Geometry check sheet. Reference: the model listing, model coordinates, mm. Face numbers are marked on the shaded views. Coordinates: 2 decimals unless noted, no trailing zeros. Loops run counter-clockwise (first coordinate to the right, second up) from the corner with the lowest first, then second, coordinate; pieces in that order, holes last.
from build123d import *

# Parameters (mm, degrees)
SKETCH1_R           = 29
SKETCH1_R_2         = 25.5
BOSS_EXTRUDE1_DEPTH = 30
CUT_EXTRUDE1_START  = -4
SKETCH2_R           = 26.983908251
SKETCH2_R_2         = 25.5
CUT_EXTRUDE1_DEPTH  = 4
BOSS_EXTRUDE2_START = 6
SKETCH3_R           = 29
BOSS_EXTRUDE2_DEPTH = 6
SKETCH4_R           = 4
CUT_EXTRUDE2_DEPTH  = 4.3
SKETCH5_R           = 25.5
SKETCH5_R_2         = 25.1
BOSS_EXTRUDE3_DEPTH = 2


with BuildPart() as part:
    # Sketch1 → Boss-Extrude1 (new body)
    with BuildSketch(Plane(origin=(0, 0, 0), x_dir=(1, 0, 0), z_dir=(0, 1, 0))):
        with Locations(Location((0, 0, 0), (0, 0, 270))):
            Circle(SKETCH1_R)
        with Locations(Location((0, 0, 0), (0, 0, 270))):
            Circle(SKETCH1_R_2, mode=Mode.SUBTRACT)
    extrude(amount=BOSS_EXTRUDE1_DEPTH)

    # Sketch2 → Cut-Extrude1 (cut)
    with BuildSketch(Plane(origin=(0, 30, 0), x_dir=(1, 0, 0), z_dir=(0, 1, 0)).offset(CUT_EXTRUDE1_START)):
        with Locations(Location((0, 0, 0), (0, 0, 270))):
            Circle(SKETCH2_R)
        with Locations(Location((0, 0, 0), (0, 0, 270))):
            Circle(SKETCH2_R_2, mode=Mode.SUBTRACT)
    extrude(amount=CUT_EXTRUDE1_DEPTH, mode=Mode.SUBTRACT)

    # Fillet1: read off the stored shape, not the designer's step
    # Fillet1 outline → Fillet1 (revolve, cut)
    with BuildSketch(Plane.XY):
        with BuildLine():
            ThreePointArc((26.983908251, 27.165934977), (27.539350545, 28.904939757), (29, 30))
            Line((29, 30), (26.983908251, 30))
            Line((26.983908251, 30), (26.983908251, 27.165934977))
        make_face()
    revolve(axis=Axis((0, 0, 0), (0, 1, 0)), mode=Mode.SUBTRACT)

    # Sketch3 → Boss-Extrude2 (add)
    with BuildSketch(Plane.XZ.offset(BOSS_EXTRUDE2_START)):
        with Locations(Location((0, 0, 0), (0, 0, 270))):
            Circle(SKETCH3_R)
    extrude(amount=-BOSS_EXTRUDE2_DEPTH)

    # Sketch4 → Cut-Extrude2 (cut)
    with BuildSketch(Plane(origin=(0, 0, 0), x_dir=(1, 0, 0), z_dir=(0, 1, 0))):
        with Locations(Location((0, 0, 0), (0, 0, 270))):
            Circle(SKETCH4_R)
    extrude(amount=-CUT_EXTRUDE2_DEPTH, mode=Mode.SUBTRACT)

    # Sketch5 → Boss-Extrude3 (add)
    with BuildSketch(Plane(origin=(0, 0, 0), x_dir=(1, 0, 0), z_dir=(0, 1, 0))):
        with Locations(Location((0, 0, 0), (0, 0, 270))):
            Circle(SKETCH5_R)
        with Locations(Location((0, 0, 0), (0, 0, 270))):
            Circle(SKETCH5_R_2, mode=Mode.SUBTRACT)
    extrude(amount=BOSS_EXTRUDE3_DEPTH)


solid = part.part
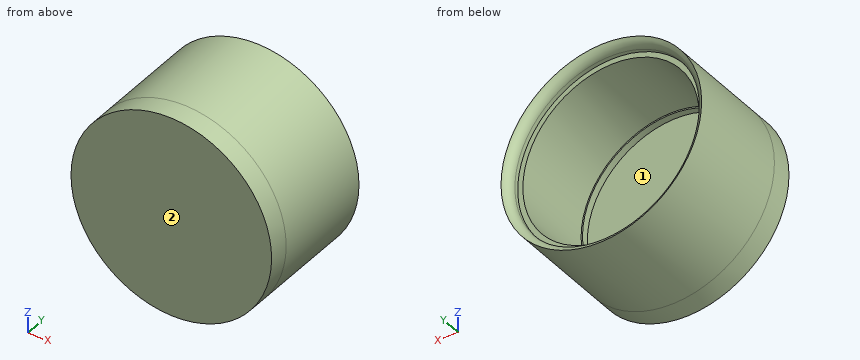
(1) Sectioned sample at A-A on z = 0. Record the cut outline in (x, y).
Findings:
outline: (-29, -6) - (29, -6) - (29, 30) arc R3 ccw to (26.98, 27.17) - (26.98, 26) - (25.5, 26) - (25.5, 2) - (25.1, 2) - (25.1, 0) - (4, 0) - (4, -4.3) - (-4, -4.3) - (-4, 0) - (-25.1, 0) - (-25.1, 2) - (-25.5, 2) - (-25.5, 26) - (-26.98, 26) - (-26.98, 27.17) arc R3 ccw to (-29, 30) - close
(2) Gauge pin test, flat ends, axial feed: pin 1 Ø1.5 at (x, z) = (17, -8.5) entering from +Y; pin 2 Ø2.5 at (x, z) = (1, 2) entering from +Y; pin 3 Ø1 at (y, z) = (13, 19) entering from -X; pin 4 Ø8 at (x, y) = (-0.5, 10.5) entering from +Z. Record the tip position at first contact, or that the pin passes through.
Findings:
pin 1: stops at y = 0
pin 2: stops at y = -4.3
pin 3: stops at x = -22.33
pin 4: stops at z = 29
(3) Sectioned sample at C-C on y = -2. Record the cut outline in (x, z), and give its area (3 significant figures).
Findings:
outline: circle Ø58 at (0, 0); hole circle Ø8 at (0, 0)
area: 2,590 mm2
(4) Draft check along X on the marked faces 1 and 2. Enter one of: +X half, -X half, draft (parallel to the pull), parting line (faces both ways), or undercut.
Findings:
face 1: undercut
face 2: draft
(5) Scan lines: L1, parallel to Z at x = 0, y = 26.65; L2, parallel to X at y = 16.5, z = 0; L3, parallel to X at y = -2, z = 0. Record each from-to range of solid material in increasing order.
Findings:
L1: z = -29 to -26.98, 26.98 to 29
L2: x = -29 to -25.5, 25.5 to 29
L3: x = -29 to -4, 4 to 29
(6) Sectioned sample at B-B on x = 0. Record the cut outline in (y, z).
Findings:
outline: (-6, -29) - (30, -29) arc R3 ccw to (27.17, -26.98) - (26, -26.98) - (26, -25.5) - (2, -25.5) - (2, -25.1) - (0, -25.1) - (0, -4) - (-4.3, -4) - (-4.3, 4) - (0, 4) - (0, 25.1) - (2, 25.1) - (2, 25.5) - (26, 25.5) - (26, 26.98) - (27.17, 26.98) arc R3 ccw to (30, 29) - (-6, 29) - close
(7) Sectioned sample at D-D on y = 8. Record the cut outline in (x, z).
Findings:
outline: circle Ø58 at (0, 0); hole circle Ø51 at (0, 0)
